from build123d import *

# Parameters (mm, degrees)
REFRENTADO_PARA_TORNILLO_CON_CABEZA_TRON_D           = 3.4
REFRENTADO_PARA_TORNILLO_CON_CABEZA_TRON_CBORE_D     = 7
REFRENTADO_PARA_TORNILLO_CON_CABEZA_TRON_CBORE_DEPTH = 2.4
CORTAR_EXTRUIR1_DEPTH                                = 2.4


with BuildPart() as part:
    # Croquis2 → Revolución1 (revolve)
    with BuildSketch(Plane(origin=(0, 0, 0), x_dir=(1, 0, 0), z_dir=(0, 1, 0)), mode=Mode.PRIVATE) as revoluci_n1_sk:
        Polygon((0, 32.7), (20.1, 32.7), (20.1, 24), (9.5, 24), (9, 23.5), (2, 23.5), (2, 21.7), (0, 21.7), align=None)
    revolve(revoluci_n1_sk.sketch.rotate(Axis((-10.750662053, 0, 0), (1, 0, 0)), 180), axis=Axis((-10.750662053, 0, 0), (1, 0, 0)))

    # Refrentado para tornillo con cabeza troncocónica de M31 (through all)
    with Locations(Plane.ZY):
        with Locations((14.5, 25.11473671), (29, 0), (14.5, -25.11473671), (-14.5, -25.11473671), (-29, 0), (-14.5, 25.11473671)):
            CounterBoreHole(REFRENTADO_PARA_TORNILLO_CON_CABEZA_TRON_D / 2, REFRENTADO_PARA_TORNILLO_CON_CABEZA_TRON_CBORE_D / 2, REFRENTADO_PARA_TORNILLO_CON_CABEZA_TRON_CBORE_DEPTH)

    # Croquis6 → Cortar-Extruir1 (cut)
    with BuildSketch(Plane.ZY):
        with BuildLine():
            Line((29, 3.5), (32.512151574, 3.5))
            ThreePointArc((32.512151574, 3.5), (32.7, 0), (32.512151574, -3.5))
            Line((32.512151574, -3.5), (29, -3.5))
            ThreePointArc((29, -3.5), (25.5, 0), (29, 3.5))
        make_face()
        with BuildLine():
            Line((17.531088913, -23.36473671), (19.2871647, -26.406349195))
            ThreePointArc((19.2871647, -26.406349195), (16.35, -28.319030704), (13.224986874, -29.906349195))
            Line((13.224986874, -29.906349195), (11.468911087, -26.86473671))
            ThreePointArc((11.468911087, -26.86473671), (12.75, -22.083647797), (17.531088913, -23.36473671))
        make_face()
        with BuildLine():
            Line((-11.468911087, -26.86473671), (-13.224986874, -29.906349195))
            ThreePointArc((-13.224986874, -29.906349195), (-16.35, -28.319030704), (-19.2871647, -26.406349195))
            Line((-19.2871647, -26.406349195), (-17.531088913, -23.36473671))
            ThreePointArc((-17.531088913, -23.36473671), (-12.75, -22.083647797), (-11.468911087, -26.86473671))
        make_face()
        with BuildLine():
            Line((-29, -3.5), (-32.512151574, -3.5))
            ThreePointArc((-32.512151574, -3.5), (-32.7, 0), (-32.512151574, 3.5))
            Line((-32.512151574, 3.5), (-29, 3.5))
            ThreePointArc((-29, 3.5), (-25.5, 0), (-29, -3.5))
        make_face()
        with BuildLine():
            Line((-17.531088913, 23.36473671), (-19.2871647, 26.406349195))
            ThreePointArc((-19.2871647, 26.406349195), (-16.35, 28.319030704), (-13.224986874, 29.906349195))
            Line((-13.224986874, 29.906349195), (-11.468911087, 26.86473671))
            ThreePointArc((-11.468911087, 26.86473671), (-12.75, 22.083647797), (-17.531088913, 23.36473671))
        make_face()
        with BuildLine():
            Line((11.468911087, 26.86473671), (13.224986874, 29.906349195))
            ThreePointArc((13.224986874, 29.906349195), (16.35, 28.319030704), (19.2871647, 26.406349195))
            Line((19.2871647, 26.406349195), (17.531088913, 23.36473671))
            ThreePointArc((17.531088913, 23.36473671), (12.75, 22.083647797), (11.468911087, 26.86473671))
        make_face()
    extrude(amount=-CORTAR_EXTRUIR1_DEPTH, mode=Mode.SUBTRACT)


solid = part.part
Input: part model. Units: mm. Frame: model coordinates. A direction names the side the tool comes from. Coordinates: 2 decimals unless noted, no trailing zeros. Order: outer loops, then holes, each group sorted by start corner. A loop starts at its lowest first (then second) coordinate and runs counter-clockwise, first axis right, second up. Notation, with made-up numbers: M 18.25,27 L 29.25,27 A8 cw 29.25,41 Z; hole C 44,67 d5. An arc over 180 degrees is marked long. Answer as CSV lines item,"result".
1. Material intervals for line 1 (Y direction, x = 14.5, z = -14.5); line 2 (Z direction, x = 17.25, y = -25); line 3 (Z direction, x = 11, y = 3), sorted ascending. Write a range as from..to.
Reported:
line 1,"-29.31..-26.81, -23.41..-19.12, 19.12..23.41, 26.81..29.31"
line 2,"-21.08..-16.2, -12.8..12.8, 16.2..21.08"
line 3,"-32.56..-23.81, 23.81..32.56"
2. Access query for faces 5 (the flat face through (1, -3.5, -31)), 6 (the flat face through (1.183, 24.864, -18.397)), 7 (the flat face through (2.4, -27, -16)). Directions: +Z, -Z, +X, -X, +Y, -Y. A direction counts if a zero-diameter tool reaches every point of the face in a straight line with its end or side. Return the directions, or none.
Reported:
face 5,"-Z, -X"
face 6,"-X, +Y"
face 7,"-X"
3. Section D-D (y = 28.5). Return the cut outline in (x, z).
Reported:
outline,"M 0,-12.41 L 2.4,-12.41 L 2.4,-16.03 L 20.1,-16.03 L 20.1,16.03 L 2.4,16.03 L 2.4,12.41 L 0,12.41 Z"
4. Pull-direction query (Z, two-part tool) for faces 1 (the cylindrical face through (1.183, -22.123, 12.684)), 2 (the cylindrical face through (1.2, -0.1, 25.5)), 3 (the flat face through (1, -3.5, 31)), 4 (the flat face through (1.18, 28.41, -12.36)); classes: released by +Z, released by -Z, zero draft, split by the parting line, or undercut.
Reported:
face 1,"undercut"
face 2,"released by +Z"
face 3,"zero draft"
face 4,"released by -Z"
5. First-contact query: P1, Ø6, axis at x = 3.5, z = 12.5, coming from the -Y side; P2, Ø7.5, axis at y = -1.5, z = -28, coming from the -X side; P3, Ø4.5, axis at y = 0, z = -29, coming from the -X side; P4, Ø2.5, axis at x = 1.5, z = 30.5, coming from the -Y side. Flat tips, straight axial feed; report the tip coordinate or a pass-through.
Reported:
P1,"y = -31.29"
P2,"x = 0"
P3,"x = 2.4"
P4,"y = -14.62"
6. Section C-C (x = 13.5). Return the cut outline in (y, z), then the cut area to 3 significant figures.
Reported:
outline,"C 0,0 d65.4; hole C -25.11,-14.5 d3.4; hole C -25.11,14.5 d3.4; hole C 0,0 d48; hole C 0,-29 d3.4; hole C 0,29 d3.4; hole C 25.11,-14.5 d3.4; hole C 25.11,14.5 d3.4"
area,"1,500 mm2"
7. Section A-A (y = 0). Return the cut outline in (x, z), then the cut area to 3 significant figures.
Reported:
outline,"M 0,-25.5 L 2.4,-25.5 L 2.4,-27.3 L 20.1,-27.3 L 20.1,-24 L 9.5,-24 L 9,-23.5 L 2,-23.5 L 2,-21.7 L 0,-21.7 Z; M 0,21.7 L 2,21.7 L 2,23.5 L 9,23.5 L 9.5,24 L 20.1,24 L 20.1,27.3 L 2.4,27.3 L 2.4,25.5 L 0,25.5 Z; M 2.4,-32.7 L 20.1,-32.7 L 20.1,-30.7 L 2.4,-30.7 Z; M 2.4,30.7 L 20.1,30.7 L 20.1,32.7 L 2.4,32.7 Z"
area,"211 mm2"
8. Section B-B (z = 0). Return the cut outline in (x, y), then the cut area to 3 significant figures.
Reported:
outline,"M 0,-32.7 L 20.1,-32.7 L 20.1,-24 L 9.5,-24 L 9,-23.5 L 2,-23.5 L 2,-21.7 L 0,-21.7 Z; M 0,21.7 L 2,21.7 L 2,23.5 L 9,23.5 L 9.5,24 L 20.1,24 L 20.1,32.7 L 0,32.7 Z"
area,"366 mm2"
